Can you work these out from the model? Positions are in its coordinate system, mm. A direction names the side the tool comes from. Coordinates: 2 decimals unless noted, no trailing zeros. Write each loop counter-clockwise with the first axis right and the second up, starting at its lowest first coordinate (ties: lowest second). Pieces come first, ordered by that corner, then holes. Notation, with made-up numbers: (-26, 81.5) -> (3, 81.5) arc R32 cw to (3, 114.5) -> close; hole circle Ø7 at (18.25, -33.5). An arc over 180 degrees is marked (long way). Use one line per item in the form item = value.
Autodesk Inventor part; units mm, degrees
ref_plane "作業平面1" through (-18, 70, -30) normal (0, -1, 0) x (1, 0, 0)
ref_plane "YZ Plane" through (0, 0, 0) normal (1, 0, 0) x (0, 1, 0)
ref_plane "XZ Plane" through (0, 0, 0) normal (0, 1, 0) x (-1, 0, 0)
sketch "スケッチ1" plane through (0, 0, 0) normal (1, 0, 0) x (0, 1, 0)
  line L0 (0, 0) -> (36.4832, 0)
  line L1 (36.4832, 0) -> (57.4894, -30)
  line L2 (57.4894, -30) -> (0, -30)
  line L3 (0, -30) -> (0, 0)
  dimension "d0" = 35
  dimension "d1" = 36.4832
  dimension "d2" = 30
extrude "押し出し1" add sketch "スケッチ1" along normal mid plane 36
ref_plane "作業平面1" through (-18, 70, -30) normal (0, -1, 0) x (1, 0, 0)
sketch "スケッチ3" plane through (-18, 70, -30) normal (0, -1, 0) x (1, 0, 0)
  line L0 (0, 0) -> (36, 0)
  line L1 (0, 30) -> (0, 0)
  line L2 (36, 0) -> (36, 30)
  point P0 (18, 30)
  point P1 (8, 10)
  point P2 (28, 10)
  dimension "d11" = 10
  dimension "d12" = 8
  dimension "d13" = 8
  dimension "d14" = 10
hole "穴1" at (-10, 70, -20) at (10, 70, -20) direction (0, -1, 0) diameter 5.5 end through all counterbore diameter 10 counterbore depth 40.5
sketch "スケッチ4" plane through (-18, 36.4832, 0) normal (0, 0.8192, 0.5736) x (1, 0, 0)
  line L0 (18, 10) -> (18, 10)
  line L1 (18, 10) -> (18, 26.6232)
  line L2 (18, 26.6232) -> (18, 26.6232)
  line L3 (18, 26.6232) -> (18, 10)
  line L4 (0, 36.6232) -> (36, 36.6232)
  line L5 (0, 0) -> (36, 0)
  line L6 (0, 0) -> (0, 36.6232)
  line L7 (36, 36.6232) -> (36, 0)
  point P0 (18, -20.9259)
  dimension "d22" = 36.6232
  dimension "d24" = 10
  dimension "d36" = 10
  dimension "d46" = 18
  dimension "d47" = 18
  dimension "d51" = 36
hole "穴2" at (0, 51.7537, -21.8085) at (0, 42.219, -8.1915) at (0, 51.7537, -21.8085) at (0, 42.219, -8.1915) direction (0, -0.8192, -0.5736) diameter 5 depth 6 tip angle 118
sketch "スケッチ5" plane through (18, 0, 0) normal (1, 0, 0) x (0, 0, -1)
  circle A0 centre (10, 10) radius 6.05
  line L0 (0, 0) -> (30, 0)
  line L1 (0, 36.4832) -> (0, 0)
  dimension "d40" = 10
  dimension "d41" = 10
  dimension "d42" = 12.1
extrude "押し出し3" cut sketch "スケッチ5" against normal through all
equation "\"d46\" = 0.5 * d51"
equation "\"d47\" = d46"
properties part number "s_base1"
Q1. Suppose I cut it at B-B (y = 14.5). Write out the boundary of the cut face in (x, z).
Return value:
outline = (-18, -30) -> (18, -30) -> (18, -14.04) -> (-18, -14.04) -> close; (-18, -5.96) -> (18, -5.96) -> (18, 0) -> (-18, 0) -> close; hole circle Ø5.5 at (-10, -20); hole circle Ø5.5 at (10, -20)
Q2. Suppose I cut it at C-C (z = -19). Write out the boundary of the cut face in (x, y), then the cut area to 3 significant figures.
Return value:
outline = (-18, 0) -> (-12.56, 0) -> (-12.56, 29.5) -> (-14.9, 29.5) -> (-14.9, 49.79) -> (-18, 49.79) -> close; (-7.44, 0) -> (7.44, 0) -> (7.44, 29.5) -> (5.1, 29.5) -> (5.1, 49.79) -> (-5.1, 49.79) -> (-5.1, 29.5) -> (-7.44, 29.5) -> close; (12.56, 0) -> (18, 0) -> (18, 49.79) -> (14.9, 49.79) -> (14.9, 29.5) -> (12.56, 29.5) -> close
area = 1,090 mm2
Q3. Thinking about a two-plate mould opening in Z: for faces 1 (the flat face through (0, 0, -15)), 2 (the flat face through (0, 29, -30)), 3 (the flat face through (-7.8, 29.5, -17.8)), which applies, released by +Z, released by -Z, zero draft, split by the parting line, or undercut?
Return value:
face_1 = zero draft
face_2 = released by -Z
face_3 = undercut
Q4. Will these pins go through, and if not, where does the flat tip stop? pin 1 (3 mm diameter, centred on x = 10, z = -10, fed in from +Y); pin 2 (9.5 mm diameter, centred on y = 10, z = -10, fed in from +X); pin 3 (8 mm diameter, centred on x = -9.5, z = -5.5, fed in from +Y); pin 4 (7 mm diameter, centred on x = -10, z = -20, fed in from +Y).
Return value:
pin_1 = 44.54
pin_2 = through
pin_3 = 43.14
pin_4 = 29.5
Q5. Suppose I cut it at A-A (x = -10). Write out the boundary of the cut face in (y, z).
Return value:
outline = (0, -30) -> (57.49, -30) -> (53.99, -25) -> (29.5, -25) -> (29.5, -22.75) -> (0, -22.75) -> close; (0, -17.25) -> (29.5, -17.25) -> (29.5, -15) -> (46.99, -15) -> (36.48, 0) -> (0, 0) -> close; hole circle Ø12.1 at (10, -10)
Q6. If I drill on line 1 (X direction, y = 6, z = -20); line 2 (X direction, y = 44, z = -20); line 3 (Y direction, x = 11, z = -6.5), over which ranges is the centre line in solid material (lowest first)? Write a range as from..to.
Return value:
line_1 = -18..-12.75, -7.25..7.25, 12.75..18
line_2 = -18..-15, -5..5, 15..18
line_3 = 0..5.07, 14.93..41.03
Q7. For faces 4 (the cylindrical face through (10, 39, -25)), 5 (the conical face through (0.13, 45.584, -25.623)), 6 (the cylindrical face through (0.252, 4.094, -8.688)), which set-ups out of +Z, -Z, +X, -X, +Y, -Y let a thin tool reach every point of the face, with its end or its side?
Return value:
face_4 = +Y
face_5 = none
face_6 = +X, -X
Q8. Suppose I cut it at D-D (y = 30.5). Write out the boundary of the cut face in (x, z).
Return value:
outline = (-18, -30) -> (18, -30) -> (18, 0) -> (-18, 0) -> close; hole circle Ø10 at (-10, -20); hole circle Ø10 at (10, -20)
